from build123d import *

# Parameters (mm, degrees)
BOSS_EXTRUDE1_DEPTH = 98
CUT_EXTRUDE1_REACH  = 40.016
SKETCH2_W           = 11
SKETCH2_H           = 10
SKETCH4_W           = 11
SKETCH4_H           = 10
BOSS_EXTRUDE2_DEPTH = 1.016
FILLET2_R           = 1
CUT_EXTRUDE2_REACH  = 40.016
SKETCH6_R           = 1.4224
FILLET4_R           = 1
CUT_EXTRUDE4_REACH  = 91.728
SKETCH8_W           = 20
SKETCH8_H           = 8.016
CUT_EXTRUDE5_REACH  = 90.79
SKETCH9_W           = 15
SKETCH9_H           = 22
CUT_EXTRUDE6_REACH  = 40.016
SKETCH11_W          = 15
SKETCH11_H          = 10
BOSS_EXTRUDE4_DEPTH = 1.016
CUT_EXTRUDE7_REACH  = 79.143


with BuildPart() as part:
    # Sketch1 → Boss-Extrude1 (new body)
    with BuildSketch(Plane.XY):
        Polygon((0, 0), (-5.457086284, 37), (-87.707086284, 37), (-88.723086284, 37), (-88.723086284, 48.016), (-87.707086284, 48.016), (-87.707086284, 38.016), (-4.579943874, 38.016), (1.005126579, 0.148244932), align=None)
    extrude(amount=BOSS_EXTRUDE1_DEPTH)

    # Sketch2 → Cut-Extrude1 (cut, up to next)
    with BuildSketch(Plane(origin=(0, 38.016, 0), x_dir=(1, 0, 0), z_dir=(0, 1, 0)), mode=Mode.PRIVATE) as cut_extrude1_sk1:
        with Locations((-42.399943874, -5)):
            Rectangle(SKETCH2_W, SKETCH2_H)
    cut_extrude1_tool1 = extrude(cut_extrude1_sk1.sketch, amount=-CUT_EXTRUDE1_REACH, mode=Mode.PRIVATE) & part.part
    add(cut_extrude1_tool1.solids().sort_by_distance((-42.399944, 38.016, 5))[0], mode=Mode.SUBTRACT)
    # Sketch2 → Cut-Extrude1 (cut, up to next)
    with BuildSketch(Plane(origin=(0, 38.016, 0), x_dir=(1, 0, 0), z_dir=(0, 1, 0)), mode=Mode.PRIVATE) as cut_extrude1_sk2:
        with Locations((-42.399943874, -93)):
            Rectangle(SKETCH2_W, SKETCH2_H)
    cut_extrude1_tool2 = extrude(cut_extrude1_sk2.sketch, amount=-CUT_EXTRUDE1_REACH, mode=Mode.PRIVATE) & part.part
    add(cut_extrude1_tool2.solids().sort_by_distance((-42.399944, 38.016, 93))[0], mode=Mode.SUBTRACT)

    # Sketch4 → Boss-Extrude2 (add)
    with BuildSketch(Plane(origin=(0, 0, 10), x_dir=(-1, 0, 0), z_dir=(0, 0, -1))):
        with Locations((42.399943874, 43.016)):
            Rectangle(SKETCH4_W, SKETCH4_H)
        with BuildLine():
            Line((43.989943874, 40.516), (43.989943874, 42.516))
            ThreePointArc((43.989943874, 42.516), (42.399943874, 44.106), (40.809943874, 42.516))
            Line((40.809943874, 42.516), (40.809943874, 40.516))
            ThreePointArc((40.809943874, 40.516), (42.399943874, 38.926), (43.989943874, 40.516))
        make_face(mode=Mode.SUBTRACT)
    boss_extrude2 = extrude(amount=-BOSS_EXTRUDE2_DEPTH)

    # Fillet2
    fillet2_edges = [part.edges().sort_by_distance(p)[0] for p in [
        (-42.399943874, 37, 10),
    ]]
    fillet(fillet2_edges, radius=FILLET2_R)

    # Sketch6 → Cut-Extrude2 (cut, up to next)
    with BuildSketch(Plane(origin=(0, 38.016, 0), x_dir=(1, 0, 0), z_dir=(0, 1, 0)), mode=Mode.PRIVATE) as cut_extrude2_sk1:
        with Locations((-20.739943874, -49)):
            Circle(SKETCH6_R)
    cut_extrude2_tool1 = extrude(cut_extrude2_sk1.sketch, amount=-CUT_EXTRUDE2_REACH, mode=Mode.PRIVATE) & part.part
    add(cut_extrude2_tool1.solids().sort_by_distance((-20.739944, 38.016, 49))[0], mode=Mode.SUBTRACT)

    # Mirror4: Boss-Extrude2 across plane
    add(boss_extrude2.mirror(Plane.XY.offset(49)))

    # Fillet4
    fillet4_edges = [part.edges().sort_by_distance(p)[0] for p in [
        (-42.399943874, 37, 88),
    ]]
    fillet(fillet4_edges, radius=FILLET4_R)

    # Sketch8 → Cut-Extrude4 (cut, up to next)
    with BuildSketch(Plane.ZY.offset(88.723086284), mode=Mode.PRIVATE) as cut_extrude4_sk1:
        with BuildLine():
            Line((23.41, 42.516), (23.41, 40.516))
            ThreePointArc((23.41, 40.516), (25, 38.926), (26.59, 40.516))
            Line((26.59, 40.516), (26.59, 42.516))
            ThreePointArc((26.59, 42.516), (25, 44.106), (23.41, 42.516))
        make_face()
    cut_extrude4_tool1 = extrude(cut_extrude4_sk1.sketch, amount=-CUT_EXTRUDE4_REACH, mode=Mode.PRIVATE) & part.part
    add(cut_extrude4_tool1.solids().sort_by_distance((-88.723086, 41.516, 25))[0], mode=Mode.SUBTRACT)
    # Sketch8 → Cut-Extrude4 (cut, up to next)
    with BuildSketch(Plane.ZY.offset(88.723086284), mode=Mode.PRIVATE) as cut_extrude4_sk2:
        with BuildLine():
            Line((71.41, 42.516), (71.41, 40.516))
            ThreePointArc((71.41, 40.516), (73, 38.926), (74.59, 40.516))
            Line((74.59, 40.516), (74.59, 42.516))
            ThreePointArc((74.59, 42.516), (73, 44.106), (71.41, 42.516))
        make_face()
    cut_extrude4_tool2 = extrude(cut_extrude4_sk2.sketch, amount=-CUT_EXTRUDE4_REACH, mode=Mode.PRIVATE) & part.part
    add(cut_extrude4_tool2.solids().sort_by_distance((-88.723086, 41.516, 73))[0], mode=Mode.SUBTRACT)
    # Sketch8 → Cut-Extrude4 (cut, up to next)
    with BuildSketch(Plane.ZY.offset(88.723086284), mode=Mode.PRIVATE) as cut_extrude4_sk3:
        with Locations((49, 44.008)):
            Rectangle(SKETCH8_W, SKETCH8_H)
    cut_extrude4_tool3 = extrude(cut_extrude4_sk3.sketch, amount=-CUT_EXTRUDE4_REACH, mode=Mode.PRIVATE) & part.part
    add(cut_extrude4_tool3.solids().sort_by_distance((-88.723086, 44.008, 49))[0], mode=Mode.SUBTRACT)

    # Sketch9 → Cut-Extrude5 (cut, up to next)
    with BuildSketch(Plane(origin=(1.005126579, 0.148244932, 0), x_dir=(0, 0, -1), z_dir=(0.989297814, 0.145910366, 0)), mode=Mode.PRIVATE) as cut_extrude5_sk1:
        with Locations((-49, 24.27740699)):
            Rectangle(SKETCH9_W, SKETCH9_H)
    cut_extrude5_tool1 = extrude(cut_extrude5_sk1.sketch, amount=-CUT_EXTRUDE5_REACH, mode=Mode.PRIVATE) & part.part
    add(cut_extrude5_tool1.solids().sort_by_distance((-2.537199, 24.165831, 49))[0], mode=Mode.SUBTRACT)

    # Sketch10 → Cut-Extrude6 (cut, up to next)
    with BuildSketch(Plane(origin=(0, 38.016, 0), x_dir=(1, 0, 0), z_dir=(0, 1, 0)), mode=Mode.PRIVATE) as cut_extrude6_sk1:
        Polygon((-4.579943874, -56.5), (-11.579943874, -56.5), (-11.579943874, -41.5), (-4.579943874, -41.5), (-1.579943874, -41.5), (-1.579943874, -56.5), align=None)
    cut_extrude6_tool1 = extrude(cut_extrude6_sk1.sketch, amount=-CUT_EXTRUDE6_REACH, mode=Mode.PRIVATE) & part.part
    add(cut_extrude6_tool1.solids().sort_by_distance((-6.579944, 38.016, 49))[0], mode=Mode.SUBTRACT)

    # Sketch11 → Boss-Extrude4 (add)
    with BuildSketch(Plane(origin=(-11.579943874, 0, 0), x_dir=(0, 0, -1), z_dir=(1, 0, 0))):
        with Locations((-49, 43.016)):
            Rectangle(SKETCH11_W, SKETCH11_H)
    extrude(amount=-BOSS_EXTRUDE4_DEPTH)

    # Sketch12 → Cut-Extrude7 (cut, up to next)
    with BuildSketch(Plane(origin=(-11.579943874, 0, 0), x_dir=(0, 0, -1), z_dir=(1, 0, 0)), mode=Mode.PRIVATE) as cut_extrude7_sk1:
        with BuildLine():
            Line((-50.59, 42.516), (-50.59, 40.516))
            ThreePointArc((-50.59, 40.516), (-49, 38.926), (-47.41, 40.516))
            Line((-47.41, 40.516), (-47.41, 42.516))
            ThreePointArc((-47.41, 42.516), (-49, 44.106), (-50.59, 42.516))
        make_face()
    cut_extrude7_tool1 = extrude(cut_extrude7_sk1.sketch, amount=-CUT_EXTRUDE7_REACH, mode=Mode.PRIVATE) & part.part
    add(cut_extrude7_tool1.solids().sort_by_distance((-11.579944, 41.516, 49))[0], mode=Mode.SUBTRACT)


solid = part.part
Input: part model. Units: mm. Frame: model coordinates. A direction names the side the tool comes from. Give positions to 0.01 mm unless a question says otherwise; leave off trailing zeros. Order: outer loops, then holes, each group sorted by start corner. A loop starts at its lowest first (then second) coordinate and runs counter-clockwise, first axis right, second up. Notation, with made-up numbers: (28, 48) - (60, 48) arc R22 ccw to (60, 84) - close; hole circle Ø9 at (74.5, 13). An arc over 180 degrees is marked (long way). Write each question's results on one line, items separated by ' | '.
Item 1: Material intervals for line 1 along X through (y, z) = (39, 51); line 2 along Y through (x, z) = (-82, 76); line 3 along X through (y, z) = (42, 63.5), sorted ascending.
A:
line 1: x = -88.72 to -87.71, -12.6 to -11.58 | line 2: y = 37 to 38.02 | line 3: x = -88.72 to -87.71
Item 2: Access query for faces 1 (the flat face through (-12.596, 43, 51)), 2 (the flat face through (-41, 44, 86.984)), 3 (the flat face through (-48, 37, 48)), 4 (the flat face through (-11.58, 43, 51)). Directions: +Z, -Z, +X, -X, +Y, -Y. A direction counts if a zero-diameter tool reaches every point of the face in a straight line with its end or side. Return the directions, or none.
A:
face 1: +Z, -Z, +Y | face 2: +X, +Y | face 3: +Z, -Z, -X, -Y | face 4: +X, +Y, -Y
Item 3: Draft query along Z for faces 5 (the flat face through (-3.9, 27.5, 41.5)), 6 (the flat face through (-74.3, 37.6, 98)), 7 (the flat face through (-87.707, 39.8, 48.3)). Return one class per face: released by +Z, released by -Z, zero draft, split by the parting line, or undercut.
A:
face 5: undercut | face 6: released by +Z | face 7: zero draft
Item 4: Section C-C (z = 25). Return loops of the section in (x, y).
A:
outline: (-88.72, 37) - (-5.46, 37) - (0, 0) - (1.01, 0.15) - (-4.58, 38.02) - (-87.71, 38.02) - (-87.71, 38.93) - (-88.72, 38.93) - close; (-88.72, 44.11) - (-87.71, 44.11) - (-87.71, 48.02) - (-88.72, 48.02) - close
Item 5: Section A-A (x = -7). Return loops of the section in (y, z).
A:
outline: (37, 0) - (38.02, 0) - (38.02, 41.5) - (37, 41.5) - close; (37, 56.5) - (38.02, 56.5) - (38.02, 98) - (37, 98) - close
Item 6: Contact query for flat-ended pins moving along their axis: pin 1 Ø10 at (y, z) = (35, 72.5) entering from +X; pin 2 Ø5 at (x, y) = (-44.5, 44) entering from +Z; pin 3 Ø5 at (y, z) = (43, 50) entering from -X. Output: stop coordinate, or through.
A:
pin 1: stops at x = -3.4 | pin 2: stops at z = 88 | pin 3: stops at x = -12.6
Item 7: Section B-B (z = 49). Return loops of the section in (x, y), and give its area (3 significant figures).
A:
outline: (-88.72, 37) - (-22.16, 37) - (-22.16, 38.02) - (-87.71, 38.02) - (-87.71, 40) - (-88.72, 40) - close; (-19.32, 37) - (-11.58, 37) - (-11.58, 38.93) - (-12.6, 38.93) - (-12.6, 38.02) - (-19.32, 38.02) - close; (-12.6, 44.11) - (-11.58, 44.11) - (-11.58, 48.02) - (-12.6, 48.02) - close; (-1.94, 13.14) - (0, 0) - (1.01, 0.15) - (-0.93, 13.28) - close | area: 95.9 mm^2
Item 8: Section D-D (x = -74). Return loops of the section in (y, z).
A:
outline: (37, 0) - (38.02, 0) - (38.02, 98) - (37, 98) - close
